Work out the finished part from the listing and answer in its coordinate system (mm). Face numbers are marked on the shaded views. Coordinates: 2 decimals unless noted, no trailing zeros. Order: outer loops, then holes, each group sorted by start corner. A loop starts at its lowest first (then second) coordinate and runs counter-clockwise, first axis right, second up. Notation, with made-up numbers: (41.25, 55) -> (71.25, 55) arc R7 cw to (71.25, 63) -> close; hole circle Ø10 at (10.5, 56). An arc over 180 degrees is marked (long way). Answer as CSV lines item,"result". Start each with the question number.
Item 1: Each of these flat-tipped pins is pushed along its axis until it touches: pin 1 Ø2 at (y, z) = (-1.5, -0.5) entering from +X; pin 2 Ø1.1 at (x, y) = (1, -9.5) entering from +Z; pin 3 Ø1.1 at (x, y) = (-1, -10.5) entering from -Z. Where does it stop, or does it pass through?
Item 2: Straight lines are drawn through the part: L1, parallel to Y at x = 0.85, z = -1.3; L2, parallel to Y at x = 1, z = 0.3; L3, parallel to X at y = -2, z = 0.7. For each, find the intervals that lie inside material, in ascending order.
Item 3: For a pull along Z with two mould halves and no side action, classify the marked faces 1, 2 and 3 as pulls with the +Z half, pulls with the -Z half, needs draft (parallel to the pull), parting line crosses it, or undercut.
Item 4: Section A-A (x = 0) is taken. Write down the section's boundary in (y, z).
Item 5: Section C-C (z = 0) is taken. Write down the section's boundary in (x, y), then the cut area to 3 significant figures.
Item 6: Section B-B (y = -12) is taken. Write down the section's boundary in (x, z), then the cut area to 3 significant figures.
Item 7: Section D-D (x = 1.3) is taken. Write down the section's boundary in (y, z), then the cut area to 3 significant figures.
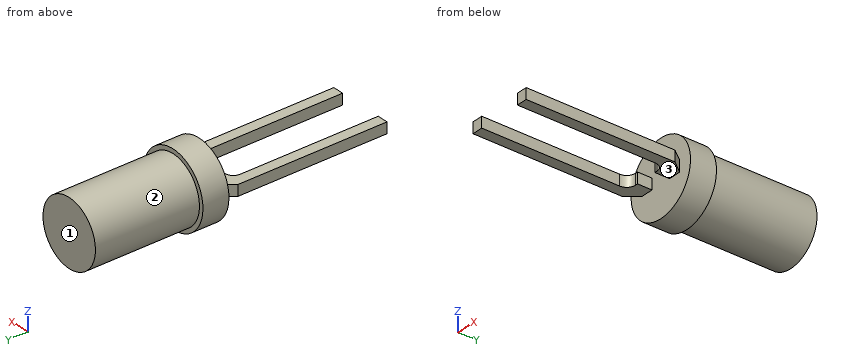
```python
from build123d import *

# Parameters (mm, degrees)
ESQUISSE1_R             = 1.5
BOSS_EXTRU_1_DEPTH      = 4.8
ESQUISSE2_R             = 1.7
BOSS_EXTRU_2_DEPTH      = 1.2
BOSS_EXTRU_3_DEPTH      = 0.25
BOSS_EXTRU_3_DEPTH_BACK = 0.25


with BuildPart() as part:
    # Esquisse1 → Boss.-Extru.1 (new body)
    with BuildSketch(Plane(origin=(0, 0, 0), x_dir=(1, 0, 0), z_dir=(0, 1, 0))):
        with Locations(Location((0, 0, 0), (0, 0, 270))):
            Circle(ESQUISSE1_R)
    extrude(amount=-BOSS_EXTRU_1_DEPTH)

    # Esquisse2 → Boss.-Extru.2 (add)
    with BuildSketch(Plane.XZ.offset(4.8)):
        with Locations(Location((0, 0, 0), (0, 0, 270))):
            Circle(ESQUISSE2_R)
    extrude(amount=BOSS_EXTRU_2_DEPTH)

    # Esquisse3 → Boss.-Extru.3 (add, two sides: drawn at the far end of the back side and taken through both)
    with BuildSketch(Plane.XY.offset(-BOSS_EXTRU_3_DEPTH_BACK)):
        with BuildLine():
            Line((0.5, -6), (0.5, -6.672497838))
            Line((0.5, -6.672497838), (0.62, -6.672497838))
            ThreePointArc((0.62, -6.672497838), (0.902842712, -6.789655126), (1.02, -7.072497838))
            Line((1.02, -7.072497838), (1.02, -13.439637098))
            Line((1.02, -13.439637098), (1.52, -13.439637098))
            Line((1.52, -13.439637098), (1.52, -6.572497838))
            Line((1.52, -6.572497838), (1.084066682, -6))
            Line((1.084066682, -6), (0.5, -6))
        make_face()
        with BuildLine():
            Line((-1.084066682, -6), (-0.5, -6))
            Line((-0.5, -6), (-0.5, -6.672497838))
            Line((-0.5, -6.672497838), (-0.62, -6.672497838))
            ThreePointArc((-0.62, -6.672497838), (-0.902842712, -6.789655126), (-1.02, -7.072497838))
            Line((-1.02, -7.072497838), (-1.02, -13.439637098))
            Line((-1.02, -13.439637098), (-1.52, -13.439637098))
            Line((-1.52, -13.439637098), (-1.52, -6.572497838))
            Line((-1.52, -6.572497838), (-1.084066682, -6))
        make_face()
    extrude(amount=BOSS_EXTRU_3_DEPTH + BOSS_EXTRU_3_DEPTH_BACK)


solid = part.part
```
Checked values:
1,pin 1,"stops at x = 1.5"
1,pin 2,"stops at z = 0.25"
1,pin 3,"stops at z = -0.25"
2,L1,"y = -6 to -4.8"
2,L2,"y = -6 to 0"
2,L3,"x = -1.33 to 1.33"
3,face 1,"needs draft"
3,face 2,"parting line crosses it"
3,face 3,"pulls with the -Z half"
4,outline,"(-6, -1.7) -> (-4.8, -1.7) -> (-4.8, -1.5) -> (0, -1.5) -> (0, 1.5) -> (-4.8, 1.5) -> (-4.8, 1.7) -> (-6, 1.7) -> close"
5,outline,"(-1.7, -6) -> (-1.08, -6) -> (-1.52, -6.57) -> (-1.52, -13.44) -> (-1.02, -13.44) -> (-1.02, -7.07) arc R0.4 cw to (-0.62, -6.67) -> (-0.5, -6.67) -> (-0.5, -6) -> (0.5, -6) -> (0.5, -6.67) -> (0.62, -6.67) arc R0.4 cw to (1.02, -7.07) -> (1.02, -13.44) -> (1.52, -13.44) -> (1.52, -6.57) -> (1.08, -6) -> (1.7, -6) -> (1.7, -4.8) -> (1.5, -4.8) -> (1.5, 0) -> (-1.5, 0) -> (-1.5, -4.8) -> (-1.7, -4.8) -> close"
5,area,"26.4 mm^2"
6,outline,"(-1.52, -0.25) -> (-1.02, -0.25) -> (-1.02, 0.25) -> (-1.52, 0.25) -> close; (1.02, -0.25) -> (1.52, -0.25) -> (1.52, 0.25) -> (1.02, 0.25) -> close"
6,area,"0.500 mm^2"
7,outline,"(-13.44, -0.25) -> (-6.28, -0.25) -> (-6.28, 0.25) -> (-13.44, 0.25) -> close; (-6, -1.1) -> (-4.8, -1.1) -> (-4.8, -0.75) -> (0, -0.75) -> (0, 0.75) -> (-4.8, 0.75) -> (-4.8, 1.1) -> (-6, 1.1) -> close"
7,area,"13.4 mm^2"
